```python
from build123d import *

# Parameters (mm, degrees)
SKETCH1_W           = 30
SKETCH1_H           = 15
BOSS_EXTRUDE1_DEPTH = 25
BOSS_EXTRUDE2_DEPTH = 15


with BuildPart() as part:
    # Sketch1 → Boss-Extrude1 (new body)
    with BuildSketch(Plane.XY):
        with Locations((15, 7.5)):
            Rectangle(SKETCH1_W, SKETCH1_H)
    extrude(amount=BOSS_EXTRUDE1_DEPTH)

    # Sketch2 → Boss-Extrude2 (add)
    with BuildSketch(Plane(origin=(30, 0, 0), x_dir=(0, 0, -1), z_dir=(1, 0, 0))):
        Polygon((0, 15), (0, 25), (-25, 15), align=None)
    extrude(amount=-BOSS_EXTRUDE2_DEPTH)


solid = part.part
```
The listing builds one solid part. Answer for the finished solid, in the listing's coordinates (mm). A direction names the side the tool comes from. Give positions to 0.01 mm unless a question says otherwise; leave off trailing zeros. Order: outer loops, then holes, each group sorted by start corner. A loop starts at its lowest first (then second) coordinate and runs counter-clockwise, first axis right, second up. Notation, with made-up numbers: (89.25, 25.5) -> (93.25, 25.5) arc R33 cw to (93.25, 56.5) -> close; hole circle Ø4 at (75.25, 27.25). An arc over 180 degrees is marked (long way). One line per item, written item: value.
1) Find section D-D, the plane z = 20.25. Determine the outline of the cut face in (x, y), plus the area to 4 significant figures.
Reported:
outline: (0, 0) -> (30, 0) -> (30, 16.9) -> (15, 16.9) -> (15, 15) -> (0, 15) -> close
area: 478.5 mm^2
2) Find section A-A, the plane z = 23.5. Determine the outline of the cut face in (x, y), plus the area to 3 significant figures.
Reported:
outline: (0, 0) -> (30, 0) -> (30, 15.6) -> (15, 15.6) -> (15, 15) -> (0, 15) -> close
area: 459 mm^2
3) Find section B-B, the plane x = 7. Determine the outline of the cut face in (y, z).
Reported:
outline: (0, 0) -> (15, 0) -> (15, 25) -> (0, 25) -> close
4) Find section C-C, the plane y = 16. Determine the outline of the cut face in (x, z), plus the area to 4 significant figures.
Reported:
outline: (15, 0) -> (30, 0) -> (30, 22.5) -> (15, 22.5) -> close
area: 337.5 mm^2
5) Find the intervals of material crossed by line 1 (Y direction, x = 2.5, z = 11.5); line 2 (Y direction, x = 18, z = 4.5), in increasing order.
Reported:
line 1: y = 0 to 15
line 2: y = 0 to 23.2
6) Flat-ended cylindrical pins translate along their axes: P1, Ø1.5, axis at x = 21, z = 20, coming from the +Y side; P2, Ø1.5, axis at x = 26, z = 16.5, coming from the +Y side; P3, Ø12, axis at x = 4, z = 7.5, coming from the +Y side. Find the tip coordinate at first contact, or state that the pin passes through.
Reported:
P1: stops at y = 17.3
P2: stops at y = 18.7
P3: stops at y = 15
7) A tool of negligible diameter and unlimited length cuts with its end or side. For faces 1 (the flat face through (15, 8, 25)), 2 (the flat face through (7, 15, 12)), from which of +Z, -Z, +X, -X, +Y, -Y can it reach the whole face along a straight path? Write none if from no direction.
Reported:
face 1: +Z, +X, -X, +Y, -Y
face 2: +Z, -Z, -X, +Y
